from build123d import *

# Parameters (mm, degrees)
BOSS_EXTRUDE1_DEPTH = 238
SKETCH6_R           = 44.45
CUT_EXTRUDE1_DEPTH  = 78
SKETCH7_W           = 33
SKETCH7_H           = 85
CUT_EXTRUDE2_DEPTH  = 19
CUT_EXTRUDE2_TAPER  = 5
CUT_EXTRUDE3_DEPTH  = 13
BOSS_EXTRUDE2_DEPTH = 33


with BuildPart() as part:
    # Sketch5 → Boss-Extrude1 (new body)
    with BuildSketch(Plane.XY):
        with BuildLine():
            Line((-84, -43.008130888), (-84, 0))
            ThreePointArc((-84, 0), (-59.39696962, 59.39696962), (0, 84))
            Line((0, 84), (0, 28.575))
            ThreePointArc((0, 28.575), (-28.575, 0), (0, -28.575))
            Line((0, -28.575), (0, -84))
            Line((0, -84), (-13, -84))
            Line((-13, -84), (-84, -43.008130888))
        make_face()
    extrude(amount=BOSS_EXTRUDE1_DEPTH)

    # Sketch6 → Cut-Extrude1 (cut)
    with BuildSketch(Plane.XY.offset(238)):
        Circle(SKETCH6_R)
    extrude(amount=-CUT_EXTRUDE1_DEPTH, mode=Mode.SUBTRACT)

    # Sketch7 → Cut-Extrude2 (cut)
    with BuildSketch(Plane(origin=(0, 0, 0), x_dir=(0, 0, -1), z_dir=(1, 0, 0))):
        with Locations((-54.5, 43.5)):
            Rectangle(SKETCH7_W, SKETCH7_H)
    extrude(amount=-CUT_EXTRUDE2_DEPTH, taper=CUT_EXTRUDE2_TAPER, mode=Mode.SUBTRACT)

    # Sketch8 → Cut-Extrude3 (cut)
    with BuildSketch(Plane(origin=(0, 0, 0), x_dir=(0, 0, -1), z_dir=(1, 0, 0))):
        with BuildLine():
            Line((-117, -47), (66, -47))
            ThreePointArc((66, -47), (77, -58), (66, -69))
            Line((66, -69), (-117, -69))
            ThreePointArc((-117, -69), (-128, -58), (-117, -47))
        make_face()
    extrude(amount=-CUT_EXTRUDE3_DEPTH, mode=Mode.SUBTRACT)

    # Sketch9 → Boss-Extrude2 (add)
    with BuildSketch(Plane.XY.offset(238)):
        with BuildLine():
            Line((-83.014649379, 12.828405531), (-65.430668922, -0.909705656))
            Line((-65.430668922, -0.909705656), (-14.946427946, 63.707176139))
            Line((-14.946427946, 63.707176139), (-32.530408402, 77.445287327))
            ThreePointArc((-32.530408402, 77.445287327), (-66.192903303, 51.715563927), (-83.014649379, 12.828405531))
        make_face()
    extrude(amount=BOSS_EXTRUDE2_DEPTH)


solid = part.part
Check sheet for the modelled part. Datum: model origin and axes. Units: mm. A direction names the side the tool comes from. Round coordinates to 2 decimals unless told otherwise and drop trailing zeros. Write each loop counter-clockwise with the first axis right and the second up, starting at its lowest first coordinate (ties: lowest second). Pieces come first, ordered by that corner, then holes. Notation, with made-up numbers: (69, -31) -> (110, -31) arc R26 ccw to (110, 3) -> close; hole circle Ø9 at (3.5, 68.25). An arc over 180 degrees is marked (long way). Answer as CSV lines item,"result". Start each with the question number.
1) Go/stop test with flat-tipped pins: P1, Ø1, axis at x = -51.5, z = 49.5, coming from the +Y side; P2, Ø8, axis at x = -62, z = 180, coming from the +Y side; P3, Ø8, axis at x = -54.5, y = -45.5, coming from the +Z side; P4, Ø24, axis at y = -57, z = 49, coming from the +X side. Record where each tip stops, or that it passes through.
2) Section check D-D on x = -50.5. Enter the section's corners in (y, z), and give its area (3 significant figures).
3) Section check B-B on z = 131. Enter the section's corners in (x, y) (3 decimals).
4) Section check A-A on x = -24. Enter the section's corners in (y, z).
5) Section check C-C on y = 16. Enter the section's corners in (x, z).
6) Tool access check on faces 1 (the flat face through (-19, 51, 55)), 2 (the flat face through (-40.54, 30.95, 254.27)), 3 (the flat face through (-6, -47, 59)), 4 (the flat face through (-74.35, 6.06, 254.27)). Record the directions out of +Z, -Z, +X, -X, +Y, -Y that give a thin tool (end or side, any length) a straight path to the whole face; none if there is none.
7) Material ranges on line 1 (Y direction, x = -6, z = 31.5); line 2 (Z direction, x = -38, y = -59); line 3 (Z direction, x = -38, y = -13.5), recorded low to high. Write a range as from..to.
8) Release check for a two-part mould opening along Y. For faces 5 (the flat face through (-23.615, 70.48, 254.269)), 6 (the flat face through (-32, 1, 160)), 7 (the flat face through (-41, 1, 0)) record: pulls with the +Y half, pulls with the -Y half, needs draft (parallel to the pull), parting line crosses it, or undercut.
Found:
1,P1,"stops at y = 66.75"
1,P2,"stops at y = 60.76"
1,P3,"stops at z = 238"
1,P4,"stops at x = 0"
2,outline,"(-62.35, 0) -> (67.12, 0) -> (67.12, 271) -> (18.2, 271) -> (18.2, 238) -> (-62.35, 238) -> close"
2,area,"32,400 mm^2"
3,outline,"(-84, -43.008) -> (-13, -84) -> (0, -84) -> (0, -28.575) arc R28.575 cw to (0, 28.575) -> (0, 84) arc R84 ccw to (-84, 0) -> close"
4,outline,"(-77.65, 0) -> (-15.51, 0) -> (-15.51, 160) -> (-37.41, 160) -> (-37.41, 238) -> (-77.65, 238) -> close; (15.51, 0) -> (80.5, 0) -> (80.5, 238) -> (70.78, 238) -> (70.78, 271) -> (52.12, 271) -> (52.12, 238) -> (37.41, 238) -> (37.41, 160) -> (15.51, 160) -> close"
5,outline,"(-82.46, 0) -> (-23.68, 0) -> (-23.68, 160) -> (-41.47, 160) -> (-41.47, 238) -> (-52.22, 238) -> (-52.22, 271) -> (-82.46, 271) -> close"
6,face 1,"+X, +Y"
6,face 2,"+Z, +X, -Y"
6,face 3,"-Z, +X"
6,face 4,"+Z, -X, -Y"
7,line 1,"y = -84..-69, -47..-27.94, 27.94..83.79"
7,line 2,"z = 0..238"
7,line 3,"z = 0..160"
8,face 5,"pulls with the +Y half"
8,face 6,"undercut"
8,face 7,"needs draft"
